from build123d import *

# Parameters (mm, degrees)
F1_DEPTH = 76.2
F2_R     = 66.9441745007
F2_R_2   = 15.875
F3_DEPTH = 50.8
F5_DEPTH = 137.16


# Not quite as in the source:
# - a feature names something its author has since deleted; it is built from what else it names


with BuildPart() as f1:
    # F0 (on Right) → F1 (new body)
    with BuildSketch(Plane.YZ):
        with BuildLine():
            Line((169.7282094477, 24.1148148653), (23.9315970236, 72.344444596))
            ThreePointArc((23.9315970236, 72.344444596), (-76.2, 0), (23.9315970236, -72.344444596))
            Line((23.9315970236, -72.344444596), (169.7282094477, -24.1148148653))
            ThreePointArc((169.7282094477, -24.1148148653), (187.1510104398, 0), (169.7282094477, 24.1148148653))
        make_face()
    extrude(amount=F1_DEPTH)

    # F2 (on face) → F3 (cut)
    with BuildSketch(Plane.YZ.offset(76.2)):
        Circle(F2_R)
        with Locations((161.7510104398, 0)):
            Circle(F2_R_2)
    extrude(amount=-F3_DEPTH, mode=Mode.SUBTRACT)

    # F4 (on Top) → F5 (cut, symmetric)
    with BuildSketch(Plane.XY):
        with BuildLine():
            add(Edge.make_bspline(
                [(76.2, 0), (69.7670128122, 106.6320095463), (15.5509841332, 89.3209706266), (33.872663393, 196.783595894), (-4.8366077244, 199.8663842678)],
                knots=[0, 0, 0, 0, 0.5611625531, 1, 1, 1, 1], degree=3))
            Line((76.2, 0), (76.2, 199.8663842678))
            Line((76.2, 199.8663842678), (-4.8366077244, 199.8663842678))
        make_face()
    extrude(amount=F5_DEPTH, both=True, mode=Mode.SUBTRACT)


solid = f1.part
Build history of the part. All positions in model axes, mm. A direction names the side the tool comes from. Give positions to 0.01 mm unless a question says otherwise; leave off trailing zeros. Write each loop counter-clockwise with the first axis right and the second up, starting at its lowest first coordinate (ties: lowest second). Pieces come first, ordered by that corner, then holes. Notation, with made-up numbers: (15, 3) - (30, 3) arc R10 cw to (30, 14) - close; hole circle Ø3 at (-22, -14). An arc over 180 degrees is marked (long way). Use one line per item in the form item = value. Start each with the question number.
1. Probe line 1 (Y direction, x = 28, z = 0); line 2 (X direction, y = 25.5, z = 27); line 3 (Y direction, x = 50, z = -6.5). List the from-to ranges inside material, lowest first. Write a range as [from, to].
2. Band-saw the part on B-B on y = -4.5. Write the cut outline in (x, z), plus the area to 3 significant figures.
3. 3-axis set-ups, long thin cutter, end or side, ignore diameter. For faces 1 (the face through (37.567, -76.173, 2.016)), 2 (the face through (26.869, 145.884, 0.507)): which of +Z, -Z, +X, -X, +Y, -Y reach the whole face in a straight line?
4. Two-plate mould, pull along Y, no slides. Class faces 3 (the face through (0, 24, 1)), 4 (the face through (9.921, 187.147, -0.445)), 5 (the face through (25.4, -1, 1)): released by +Y, released by -Y, zero draft, split by the parting line, or undercut.
5. Band-saw the part on A-A on x = 6.5. Write the cut outline in (y, z).
6. Drop flat-ended pins along their axis: pin 1 Ø10 at (x, z) = (61.5, 37.5) entering from -Y; pin 2 Ø2 at (x, y) = (54.5, 19) entering from +Z; pin 3 Ø4 at (x, z) = (62.5, 52.5) entering from -Y. Give the stop position or say it passes through.
Conclusion:
q1.line_1 = [-76.2, -66.94], [66.94, 145.88]
q1.line_2 = [0, 25.4]
q1.line_3 = [-75.92, -66.63], [66.63, 98.4]
q2.outline = (0, -76.07) - (76.2, -76.07) - (76.2, -66.79) - (25.4, -66.79) - (25.4, 66.79) - (76.2, 66.79) - (76.2, 76.07) - (0, 76.07) - close
q2.area = 4,810 mm²
q3.face_1 = +X, -X
q3.face_2 = +X
q4.face_3 = zero draft
q4.face_4 = released by +Y
q4.face_5 = undercut
q5.outline = (23.93, -72.34) - (169.73, -24.11) arc R25.4 ccw to (169.73, 24.11) - (23.93, 72.34) arc R76.2 ccw (long way) to start
q6.pin_1 = -68.92
q6.pin_2 = 74.04
q6.pin_3 = -57.06
